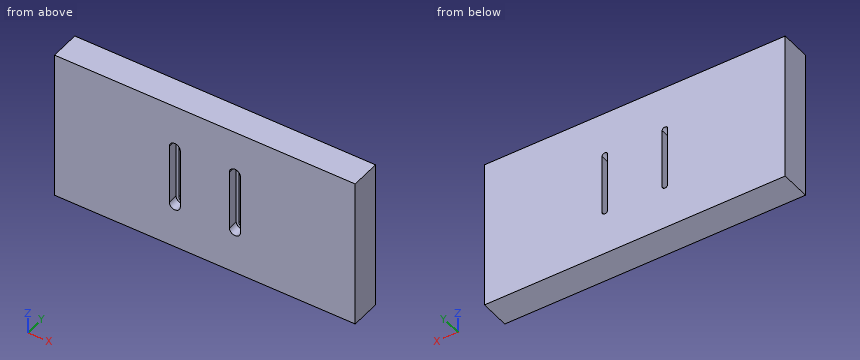
from build123d import *

# Parameters (mm, degrees)
SKETCH1_W                                        = 300
SKETCH1_H                                        = 150
BOSS_EXTRUDE1_DEPTH                              = 30
CUT_EXTRUDE2_DEPTH                               = 30
CBORE_FOR_M5_PAN_HEAD_MACHINE_SCREW1_D           = 5.5
CBORE_FOR_M5_PAN_HEAD_MACHINE_SCREW1_DEPTH       = 110
CBORE_FOR_M5_PAN_HEAD_MACHINE_SCREW1_CBORE_D     = 11
CBORE_FOR_M5_PAN_HEAD_MACHINE_SCREW1_CBORE_DEPTH = 3.7
CUT_EXTRUDE3_DEPTH                               = 10


with BuildPart() as part:
    # Sketch1 → Boss-Extrude1 (new body)
    with BuildSketch(Plane(origin=(0, 0, 0), x_dir=(1, 0, 0), z_dir=(0, 1, 0))):
        Rectangle(SKETCH1_W, SKETCH1_H)
    extrude(amount=BOSS_EXTRUDE1_DEPTH)

    # Sketch4 → Cut-Extrude2 (cut)
    with BuildSketch(Plane(origin=(0, 30, 0), x_dir=(1, 0, 0), z_dir=(0, 1, 0))):
        with BuildLine():
            Line((-32.75, -30), (-32.75, 30))
            ThreePointArc((-32.75, 30), (-30, 32.75), (-27.25, 30))
            Line((-27.25, 30), (-27.25, -30))
            ThreePointArc((-27.25, -30), (-30, -32.75), (-32.75, -30))
        make_face()
        with BuildLine():
            Line((32.75, -30), (32.75, 30))
            ThreePointArc((32.75, 30), (30, 32.75), (27.25, 30))
            Line((27.25, 30), (27.25, -30))
            ThreePointArc((27.25, -30), (30, -32.75), (32.75, -30))
        make_face()
    extrude(amount=-CUT_EXTRUDE2_DEPTH, mode=Mode.SUBTRACT)

    # CBORE for M5 Pan Head Machine Screw1
    with Locations(Plane(origin=(0, 0, 0), x_dir=(-1, 0, 0), z_dir=(0, -1, 0))):
        with Locations((30, -30), (-30, -30)):
            CounterBoreHole(CBORE_FOR_M5_PAN_HEAD_MACHINE_SCREW1_D / 2, CBORE_FOR_M5_PAN_HEAD_MACHINE_SCREW1_CBORE_D / 2, CBORE_FOR_M5_PAN_HEAD_MACHINE_SCREW1_CBORE_DEPTH, depth=CBORE_FOR_M5_PAN_HEAD_MACHINE_SCREW1_DEPTH)

    # Sketch8 → Cut-Extrude3 (cut)
    with BuildSketch(Plane.XZ):
        with BuildLine():
            Line((-24.5, 30), (-24.5, -30))
            ThreePointArc((-24.5, -30), (-30, -35.5), (-35.5, -30))
            Line((-35.5, -30), (-35.5, 30))
            ThreePointArc((-35.5, 30), (-30, 35.5), (-24.5, 30))
        make_face()
        with BuildLine():
            Line((24.5, 30), (24.5, -30))
            ThreePointArc((24.5, -30), (30, -35.5), (35.5, -30))
            Line((35.5, -30), (35.5, 30))
            ThreePointArc((35.5, 30), (30, 35.5), (24.5, 30))
        make_face()
    extrude(amount=-CUT_EXTRUDE3_DEPTH, mode=Mode.SUBTRACT)


solid = part.part
Read the model definition and answer for the solid it produces. Units are mm, in the model's axes. Give positions to 0.01 mm unless a question says otherwise; leave off trailing zeros. Write each loop counter-clockwise with the first axis right and the second up, starting at its lowest first coordinate (ties: lowest second). Pieces come first, ordered by that corner, then holes. Notation, with made-up numbers: (10, 76) - (19, 76) arc R22 ccw to (19, 115) - close; hole circle Ø9 at (2, -31.75). An arc over 180 degrees is marked (long way). Answer in a Markdown table with one row per item. Add a question column.
Item 1: Section B-B, the plane z = -0.5 is taken. Write down the section's boundary in (x, y).
Item 2: A flat-ended cylindrical pin translates along its axis: P1, Ø10, axis at x = -63, z = -45.5, coming from the -Y side. Find the tip coordinate at first contact, or state that the pin passes through.
Item 3: Section A-A, the plane x = 30 is taken. Write down the section's boundary in (y, z).
Item 4: Find the intervals of material crossed by L1, parallel to X at y = 5.5, z = 16; L2, parallel to X at y = 25.75, z = -22.5; L3, parallel to Z at x = 27, y = 2.5, in increasing order.
Item 5: Section C-C, the plane y = 22.5 is taken. Write down the section's boundary in (x, z).
Recorded:
| question | item | result |
|---|---|---|
| 1 | outline | (-150, 0) - (-35.5, 0) - (-35.5, 10) - (-32.75, 10) - (-32.75, 30) - (-150, 30) - close; (-27.25, 10) - (-24.5, 10) - (-24.5, 0) - (24.5, 0) - (24.5, 10) - (27.25, 10) - (27.25, 30) - (-27.25, 30) - close; (32.75, 10) - (35.5, 10) - (35.5, 0) - (150, 0) - (150, 30) - (32.75, 30) - close |
| 2 | P1 | stops at y = 0 |
| 3 | outline | (0, -75) - (30, -75) - (30, -32.75) - (10, -32.75) - (10, -35.5) - (0, -35.5) - close; (0, 35.5) - (10, 35.5) - (10, 32.75) - (30, 32.75) - (30, 75) - (0, 75) - close |
| 4 | L1 | x = -150 to -35.5, -24.5 to 24.5, 35.5 to 150 |
| 4 | L2 | x = -150 to -32.75, -27.25 to 27.25, 32.75 to 150 |
| 4 | L3 | z = -75 to -34.61, 34.61 to 75 |
| 5 | outline | (-150, -75) - (150, -75) - (150, 75) - (-150, 75) - close; hole (-32.75, -30) arc R2.75 ccw to (-27.25, -30) - (-27.25, 30) arc R2.75 ccw to (-32.75, 30) - close; hole (27.25, -30) arc R2.75 ccw to (32.75, -30) - (32.75, 30) arc R2.75 ccw to (27.25, 30) - close |
